Check sheet for the modelled part. Datum: model origin and axes. Units: mm. Round coordinates to 2 decimals unless told otherwise and drop trailing zeros. One line per item, written item: value.
from build123d import *

# Parameters (mm, degrees)
F2_W     = 14.801774174
F2_H     = 17.4815300852
F3_DEPTH = 12.5
F5_W     = 4.1551380418
F5_H     = 14.0508930199
F7_DEPTH = 0.5


with BuildPart() as f1:
    # F0 (on Front) → F1 (revolve)
    with BuildSketch(Plane.XZ):
        with BuildLine():
            Line((-0.4280307109, 11.4827230744), (-0.4261488038, 11.4827230744))
            add(Edge.make_bspline(
                [(-0.4261488038, 11.4827230744), (-0.556664915, 11.2998342577), (-0.6817765252, 11.007238571)],
                knots=[0.2242103955, 0.2242103955, 0.2242103955, 0.3636698207, 0.3636698207, 0.3636698207], degree=2, weights=[1, 0.9975698685, 1]))
            ThreePointArc((-0.6817765252, 11.007238571), (-0.7788007209, 10.9669177702), (-0.7377063806, 10.8702186661))
            add(Edge.make_bspline(
                [(-0.7377063806, 10.8702186661), (-4.1805245814, 2.0482402355), (-1.0087089855, -10.0145657089)],
                knots=[0.3950853549, 0.3950853549, 0.3950853549, 2.5873747735, 2.5873747735, 2.5873747735], degree=2, weights=[1, 0.4570286054, 1]))
            ThreePointArc((-1.0087089855, -10.0145657089), (-1.0611021421, -10.1053598506), (-0.9701333294, -10.1574491407))
            add(Edge.make_bspline(
                [(-0.9701333294, -10.1574491407), (-0.5208925622, -11.7775146313), (0, -11.7775146313)],
                knots=[2.610875288, 2.610875288, 2.610875288, 3.1415926536, 3.1415926536, 3.1415926536], degree=2, weights=[1, 0.9649984965, 1]))
            Line((0, -11.7775146313), (0, 11.4827230744))
            Line((0, 11.4827230744), (0, 11.7775146313))
            Line((0, 11.7775146313), (0, 12.6633324179))
            Line((0, 12.6633324179), (0, 14.7848022901))
            Line((0, 14.7848022901), (0, 16.4847507584))
            Line((0, 16.4847507584), (0, 16.7663060129))
            Line((0, 16.7663060129), (-0.5209763767, 16.7663060129))
            Line((-0.5209763767, 16.7663060129), (-0.5209763767, 16.4847507584))
            Line((-0.5209763767, 16.4847507584), (-0.3074016407, 16.4847507584))
            Line((-0.3074016407, 16.4847507584), (-0.3074016407, 14.7848022901))
            Line((-0.3074016407, 14.7848022901), (-0.419876547, 14.7848022901))
            Line((-0.419876547, 14.7848022901), (-0.419876547, 12.6633324179))
            Line((-0.419876547, 12.6633324179), (-0.4280307109, 12.6633324179))
            Line((-0.4280307109, 12.6633324179), (-0.4280307109, 11.4827230744))
        make_face()
    revolve(axis=Axis((0, 0, 0), (0, 0, -1)))

    # F2 (on Front) → F3 (cut, symmetric)
    with BuildSketch(Plane.XZ):
        with Locations((2.1127695218, 8.7407650426)):
            Rectangle(F2_W, F2_H)
    extrude(amount=F3_DEPTH, both=True, mode=Mode.SUBTRACT)

    # F4 (on Front) → F6 (revolve)
    with BuildSketch(Plane.XZ):
        Polygon((0, 0), (0, 1.129917684), (-1.5530794626, 1.129917684), (-1.5530794626, 0), (-1.5530794626, -1.129917684), (0, -1.129917684), align=None)
    revolve(axis=Axis((0, 0, -0.564958842), (0, 0, -1)))

    # F5 (on Front) → F7 (cut, symmetric)
    with BuildSketch(Plane.XZ):
        with Locations((2.0775690209, 0.1454737503)):
            Rectangle(F5_W, F5_H)
    extrude(amount=F7_DEPTH, both=True, mode=Mode.SUBTRACT)


solid = f1.part
Item 1: Material ranges on line 1 along Y through (x, z) = (0.8, -6); line 2 along X through (y, z) = (0.9, -4); line 3 along X through (y, z) = (0.65, -7.5), recorded low to high.
Result set:
line 1: -1.44 to -0.5, 0.5 to 1.44
line 2: -1.56 to 1.56
line 3: -1.33 to 1.33
Item 2: Release check for a two-part mould opening along Y. For faces 1 (the cylindrical face through (-1.55, -0.06, 0.56)), 2 (the flat face through (1, -0.5, -3)), 3 (the flat face through (-0.4, 0, 1.13)), 4 (the flat face through (0, 0, -3)) record: pulls with the +Y half, pulls with the -Y half, needs draft (parallel to the pull), parting line crosses it, or undercut.
Result set:
face 1: parting line crosses it
face 2: undercut
face 3: needs draft
face 4: undercut
Item 3: Depth check by flat-ended pin: pin 1 (1 mm diameter, centred on x = 1, z = -8.5, fed in from -Y); pin 2 (1.5 mm diameter, centred on x = -1, z = -4.5, fed in from -Y); pin 3 (0.5 mm diameter, centred on x = 0.5, y = 0, fed in from +Z). Enter the tip coordinate at first touch or a pass-through.
Result set:
pin 1: y = -1.25
pin 2: y = -1.76
pin 3: z = -6.88
